Model file for the job. Use its own axes, mm. Face numbers are marked on the shaded views. A direction names the side the tool comes from. Round coordinates to 2 decimals unless told otherwise and drop trailing zeros. Order: outer loops, then holes, each group sorted by start corner. A loop starts at its lowest first (then second) coordinate and runs counter-clockwise, first axis right, second up. Notation, with made-up numbers: (82, -2.75) -> (87, -2.75) arc R18 ccw to (87, 5.25) -> close; hole circle Ø10 at (18.25, -38). An arc over 180 degrees is marked (long way). Answer as CSV lines item,"result".
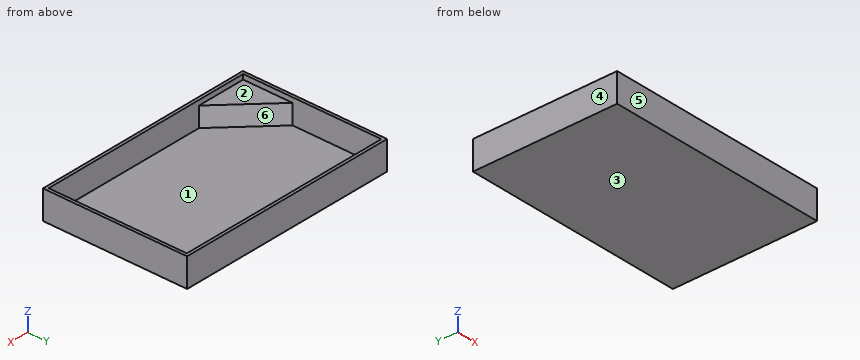
```python
from build123d import *

# Parameters (mm, degrees)
F0_W     = 90.4
F0_H     = 58.4
F0_W_2   = 88
F0_H_2   = 56
F1_DEPTH = 1.6
F2_W     = 90.4
F2_H     = 58.4
F2_W_2   = 88
F2_H_2   = 56
F3_DEPTH = 10
F5_DEPTH = 8


with BuildPart() as f1:
    # F0 (on Top) → F1 (new body)
    with BuildSketch(Plane.XY):
        Rectangle(F0_W, F0_H)
        Rectangle(F0_W_2, F0_H_2, mode=Mode.SUBTRACT)
        Rectangle(F0_W_2, F0_H_2)
    extrude(amount=F1_DEPTH)

    # F2 (on face) → F3 (join)
    with BuildSketch(Plane.XY.offset(1.6)):
        Rectangle(F2_W, F2_H)
        Rectangle(F2_W_2, F2_H_2, mode=Mode.SUBTRACT)
    extrude(amount=F3_DEPTH)

    # F4 (on face) → F5 (join)
    with BuildSketch(Plane.XY.offset(1.6)):
        Polygon((-24, -28), (-44, -8), (-44, -28), align=None)
    extrude(amount=F5_DEPTH)


solid = f1.part
```
Q1. Mould opens along X. For the marked faces 1, 2, 3 and 4 say: +X half, -X half, draft (parallel to the pull), parting line (faces both ways), or undercut.
Checks:
face 1,"undercut"
face 2,"undercut"
face 3,"draft"
face 4,"-X half"
Q2. Saw through at C-C (y = 23.5). Write the cut outline in (x, z).
Checks:
outline,"(-45.2, 0) -> (45.2, 0) -> (45.2, 11.6) -> (44, 11.6) -> (44, 1.6) -> (-44, 1.6) -> (-44, 11.6) -> (-45.2, 11.6) -> close"
Q3. Wall check: L1, parallel to X at y = 0, z = 10.5; L2, parallel to Y at x = 3, z = 4; L3, parallel to Z at x = -19.5, y = -1.5. Give the ranges that are in metal, low to high. Write a range as [from, to].
Checks:
L1,"[-45.2, -44], [44, 45.2]"
L2,"[-29.2, -28], [28, 29.2]"
L3,"[0, 1.6]"
Q4. Saw through at B-B (x = -16.5). Write the cut outline in (y, z).
Checks:
outline,"(-29.2, 0) -> (29.2, 0) -> (29.2, 11.6) -> (28, 11.6) -> (28, 1.6) -> (-28, 1.6) -> (-28, 11.6) -> (-29.2, 11.6) -> close"
Q5. Saw through at A-A (z = 6). Write the cut outline in (x, y).
Checks:
outline,"(-45.2, -29.2) -> (45.2, -29.2) -> (45.2, 29.2) -> (-45.2, 29.2) -> close; hole (-44, -8) -> (-24, -28) -> (44, -28) -> (44, 28) -> (-44, 28) -> close"
Q6. Tool access for the marked faces 5 and 6: list every direction of +Z, -Z, +X, -X, +Y, -Y with a clear straight run to the whole face (end or side of a thin tool).
Checks:
face 5,"+Z, -Z, +X, -X, -Y"
face 6,"+Z"
Q7. Flat gauge pin, fed straight in: pin 1 (10 mm diameter, centred on x = -31.5, y = -13, fed in from +Z). Where does the tip first touch, or does it go through?
Checks:
pin 1,"z = 1.6"
